Part model, mm, in its own coordinate system. Round coordinates to 2 decimals unless told otherwise and drop trailing zeros. Loops run counter-clockwise (first coordinate to the right, second up) from the corner with the lowest first, then second, coordinate; pieces in that order, holes last.
1) Band-saw the part on A-A, the plane y = 10. Write the cut outline in (x, z), then the cut area to 3 significant figures.
2) Probe line 1 (X direction, y = 0.75, z = 0); line 2 (Y direction, x = 227, z = -4.75); line 3 (Z direction, x = -196, y = 12.5). List the from-to ranges inside material, lowest first.
3) Band-saw the part on C-C, the plane x = 175. Write the cut outline in (y, z).
4) Band-saw the part on B-B, the plane x = -33. Write the cut outline in (y, z), then the cut area to 3 significant figures.
5) Drop a flat-ended pin along its axis: P1, Ø6, axis at x = 240, z = 0, coming from the +Y side. Give the stop position or say it passes through.
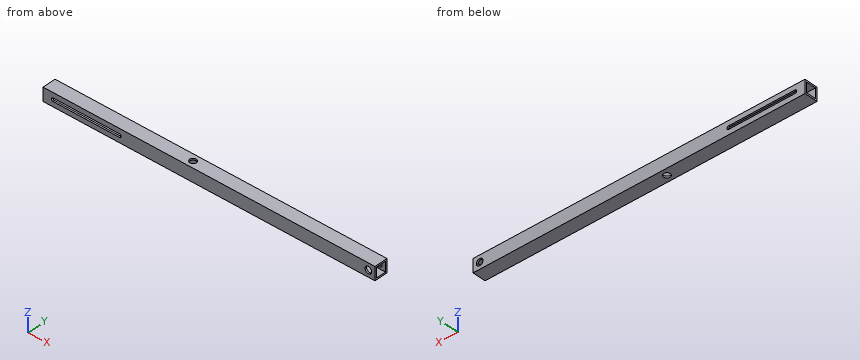
from build123d import *

# Parameters (mm, degrees)
SKETCH1_W           = 500
SKETCH1_H           = 20
BOSS_EXTRUDE1_DEPTH = 20
SKETCH6_R           = 5
CUT_EXTRUDE5_DEPTH  = 21
SKETCH8_W           = 15
SKETCH8_H           = 15
CUT_EXTRUDE7_DEPTH  = 501
CUT_EXTRUDE8_DEPTH  = 100
SKETCH10_R          = 5
CUT_EXTRUDE9_DEPTH  = 21


with BuildPart() as part:
    # Sketch1 → Boss-Extrude1 (new body)
    with BuildSketch(Plane(origin=(0, 0, 0), x_dir=(1, 0, 0), z_dir=(0, 1, 0))):
        Rectangle(SKETCH1_W, SKETCH1_H)
    extrude(amount=BOSS_EXTRUDE1_DEPTH)

    # Sketch6 → Cut-Extrude5 (cut, through all)
    with BuildSketch(Plane.XY.offset(10)):
        with Locations((-33, 10)):
            Circle(SKETCH6_R)
    extrude(amount=-CUT_EXTRUDE5_DEPTH, mode=Mode.SUBTRACT)

    # Sketch8 → Cut-Extrude7 (cut, through all)
    with BuildSketch(Plane.ZY.offset(250)):
        with Locations((0, 10)):
            Rectangle(SKETCH8_W, SKETCH8_H)
    extrude(amount=-CUT_EXTRUDE7_DEPTH, mode=Mode.SUBTRACT)

    # Sketch9 → Cut-Extrude8 (cut)
    with BuildSketch(Plane(origin=(0, 20, 0), x_dir=(1, 0, 0), z_dir=(0, 1, 0))):
        with BuildLine():
            Line((-235, 2.5), (-135, 2.5))
            ThreePointArc((-135, 2.5), (-132.5, 0), (-135, -2.5))
            Line((-135, -2.5), (-235, -2.5))
            ThreePointArc((-235, -2.5), (-237.5, 0), (-235, 2.5))
        make_face()
    extrude(amount=-CUT_EXTRUDE8_DEPTH, mode=Mode.SUBTRACT)

    # Sketch10 → Cut-Extrude9 (cut, through all)
    with BuildSketch(Plane(origin=(0, 20, 0), x_dir=(1, 0, 0), z_dir=(0, 1, 0))):
        with Locations((240, 0)):
            Circle(SKETCH10_R)
    extrude(amount=-CUT_EXTRUDE9_DEPTH, mode=Mode.SUBTRACT)


solid = part.part
Reported:
1. outline: (-250, -10) - (-38, -10) - (-38, -7.5) - (-250, -7.5) - close; (-250, 7.5) - (-38, 7.5) - (-38, 10) - (-250, 10) - close; (-28, -10) - (250, -10) - (250, -7.5) - (-28, -7.5) - close; (-28, 7.5) - (250, 7.5) - (250, 10) - (-28, 10) - close
1. area: 2,450 mm2
2. line 1: x = -250 to -237.5, -132.5 to 235, 245 to 250
2. line 2: y = 0 to 2.5, 17.5 to 20
2. line 3: z = -10 to -7.5, 7.5 to 10
3. outline: (0, -10) - (20, -10) - (20, 10) - (0, 10) - close; hole (2.5, -7.5) - (17.5, -7.5) - (17.5, 7.5) - (2.5, 7.5) - close
4. outline: (0, -10) - (5, -10) - (5, -7.5) - (2.5, -7.5) - (2.5, 7.5) - (5, 7.5) - (5, 10) - (0, 10) - close; (15, -10) - (20, -10) - (20, 10) - (15, 10) - (15, 7.5) - (17.5, 7.5) - (17.5, -7.5) - (15, -7.5) - close
4. area: 125 mm2
5. P1: passes through
